Verification items for the finished model (mm, model axes). A direction names the side the tool comes from. Round coordinates to 2 decimals unless told otherwise and drop trailing zeros. Order: outer loops, then holes, each group sorted by start corner. A loop starts at its lowest first (then second) coordinate and runs counter-clockwise, first axis right, second up. Notation, with made-up numbers: M 71,50 L 116,50 A25 cw 116,89 Z; hole C -31.75,38.5 d11. An arc over 180 degrees is marked long. One line per item, written item: value. Start each with the question number.
from build123d import *

# Parameters (mm, degrees)
ELEVATOR_SUPPORT_PULLEYS_R   = 15.875
ELEVATOR_SUPPORT_PULLEYS_R_2 = 1.016
ELEVATOR_SUPPORT_PULLEYS_W   = 6.35
ELEVATOR_SUPPORT_PULLEYS_H   = 6.35
BOSS_EXTRUDE1_DEPTH          = 6.35


with BuildPart() as part:
    # Elevator Support Pulleys → Boss-Extrude1 (new body)
    with BuildSketch(Plane(origin=(0, 0, 0), x_dir=(1, 0, 0), z_dir=(0, 1, 0))):
        with Locations(Location((0, 0, 0), (0, 0, 270))):
            Circle(ELEVATOR_SUPPORT_PULLEYS_R)
        with Locations(Location((9.398, 0, 0), (0, 0, 270))):
            Circle(ELEVATOR_SUPPORT_PULLEYS_R_2, mode=Mode.SUBTRACT)
        with Locations(Location((4.699, -8.138906745, 0), (0, 0, 270))):
            Circle(ELEVATOR_SUPPORT_PULLEYS_R_2, mode=Mode.SUBTRACT)
        with Locations(Location((-4.699, -8.138906745, 0), (0, 0, 270))):
            Circle(ELEVATOR_SUPPORT_PULLEYS_R_2, mode=Mode.SUBTRACT)
        with Locations(Location((-9.398, 0, 0), (0, 0, 270))):
            Circle(ELEVATOR_SUPPORT_PULLEYS_R_2, mode=Mode.SUBTRACT)
        with Locations(Location((-4.699, 8.138906745, 0), (0, 0, 270))):
            Circle(ELEVATOR_SUPPORT_PULLEYS_R_2, mode=Mode.SUBTRACT)
        with Locations(Location((4.699, 8.138906745, 0), (0, 0, 270))):
            Circle(ELEVATOR_SUPPORT_PULLEYS_R_2, mode=Mode.SUBTRACT)
        Rectangle(ELEVATOR_SUPPORT_PULLEYS_W, ELEVATOR_SUPPORT_PULLEYS_H, mode=Mode.SUBTRACT)
    extrude(amount=BOSS_EXTRUDE1_DEPTH)


solid = part.part
1. Section check A-A (x = 0). Record the cut outline in (y, z) (3 decimals).
2. Scan lines: line 1 along X through (y, z) = (5, 0) (3 decimals); line 2 along X through (y, z) = (5.5, 8.5); line 3 along Z through (x, y) = (-5, 5.5). Record each from-to range of solid material in increasing order.
3. Section check D-D (z = -4). Record the cut outline in (x, y), and give its area (3 significant figures).
4. Section check B-B (z = 0). Record the cut outline in (x, y) (3 decimals), and give its area (3 significant figures).
5. Draft check along X on faces 1 (the face through (4, 0, 0)), 2 (the face through (-8.39, 3.13, -0.13)), 3 (the face through (-15.497, 3.131, -3.441)). Enter one of: released by +X, released by -X, zero draft, split by the parting line, or undercut.
6. Section check C-C (y = 0.5). Record the cut outline in (x, z) (3 decimals).
7. Depth check by flat-ended pin: pin 1 (3 mm diameter, centred on y = 1.5, z = -8, fed in from +X); pin 2 (2 mm diameter, centred on x = 5, y = 4.5, fed in from +Z); pin 3 (2 mm diameter, centred on y = 2.5, z = 12, fed in from -X). Enter the tip coordinate at first touch or a pass-through.
8. Tool access check on faces 4 (the face through (-3.175, 3, 0)), 5 (the face through (4, 6.35, 0)). Record the directions out of +Z, -Z, +X, -X, +Y, -Y that give a thin tool (end or side, any length) a straight path to the whole face; none if there is none.
Geometry check:
1. outline: M 0,-15.875 L 6.35,-15.875 L 6.35,-3.175 L 0,-3.175 Z; M 0,3.175 L 6.35,3.175 L 6.35,15.875 L 0,15.875 Z
2. line 1: x = -15.875 to -10.414, -8.382 to -3.175, 3.175 to 8.382, 10.414 to 15.875
2. line 2: x = -13.41 to -5.65, -3.75 to 3.75, 5.65 to 13.41
2. line 3: z = -15.07 to -9.11, -7.17 to 7.17, 9.11 to 15.07
3. outline: M -15.36,0 L 15.36,0 L 15.36,6.35 L -15.36,6.35 Z
3. area: 195 mm²
4. outline: M -15.875,0 L -10.414,0 L -10.414,6.35 L -15.875,6.35 Z; M -8.382,0 L -3.175,0 L -3.175,6.35 L -8.382,6.35 Z; M 3.175,0 L 8.382,0 L 8.382,6.35 L 3.175,6.35 Z; M 10.414,0 L 15.875,0 L 15.875,6.35 L 10.414,6.35 Z
4. area: 135 mm²
5. face 1: zero draft
5. face 2: undercut
5. face 3: split by the parting line
6. outline: C 0,0 d31.75; hole C -9.398,0 d2.032; hole C -4.699,-8.139 d2.032; hole C -4.699,8.139 d2.032; hole M -3.175,-3.175 L 3.175,-3.175 L 3.175,3.175 L -3.175,3.175 Z; hole C 4.699,-8.139 d2.032; hole C 4.699,8.139 d2.032; hole C 9.398,0 d2.032
7. pin 1: stops at x = 14.48
7. pin 2: stops at z = 15.36
7. pin 3: stops at x = -11.45
8. face 4: +Y, -Y
8. face 5: +Z, -Z, +X, -X, +Y
